from build123d import *

# Parameters (mm, degrees)
F1_DEPTH    = 55.5
F2_T        = 4
F2_T3_DEPTH = 63.5
F3_R        = 1.5
F3_R_2      = 5
F4_DEPTH    = 132
F6_START    = -4
F6_DEPTH    = 47.5


# Not quite as in the source:
# - a shell that OpenCascade refuses in one call is made with other operations: the cavity is built on its own and cut out


with BuildPart() as f1:
    # F0 (on Right) → F1 (new body)
    with BuildSketch(Plane.YZ):
        with BuildLine():
            Line((0, -55.0991142094), (0, 49.9008857906))
            Line((0, 49.9008857906), (-499, 49.9008857906))
            Line((-499, 49.9008857906), (-499, 20.9008857906))
            Line((-499, 20.9008857906), (-542, 20.9008857906))
            Line((-542, 20.9008857906), (-542, 49.9008857906))
            Line((-542, 49.9008857906), (-571, 49.9008857906))
            Line((-571, 49.9008857906), (-585.0227475166, 32.4236936867))
            ThreePointArc((-585.0227475166, 32.4236936867), (-589.1305886162, 10.6178817454), (-573.3100487518, -4.9409842581))
            Line((-573.3100487518, -4.9409842581), (0, -55.0991142094))
        make_face()
        with BuildLine():
            ThreePointArc((-267.5215016214, -12.4960653082), (-287.1014882349, 8.865775765), (-267.5215016214, 30.2276168381))
            ThreePointArc((-267.5215016214, 30.2276168381), (-265.5317159892, 30.3083194328), (-263.5430244658, 30.2040803041))
            Line((-263.5430244658, 30.2040803041), (-227.1501212267, 29.9887811395))
            ThreePointArc((-227.1501212267, 29.9887811395), (-226.7168570765, 29.9902909304), (-226.2836411156, 29.983655073))
            ThreePointArc((-226.2836411156, 29.983655073), (-210.3577454889, 23.0383320758), (-203.8081448594, 6.9456506758))
            ThreePointArc((-203.8081448594, 6.9456506758), (-210.3577454889, -9.1470307242), (-226.2836411156, -16.0923537213))
            ThreePointArc((-226.2836411156, -16.0923537213), (-228.8553111139, -16.012257226), (-231.40202441, -15.6459876318))
            Line((-231.40202441, -15.6459876318), (-267.5215016214, -12.4960653082))
        make_face(mode=Mode.SUBTRACT)
        with BuildLine():
            ThreePointArc((-112.6117591226, 30.1063306123), (-92.6236860119, 21.9492705288), (-84.3273722818, 2.0185938124))
            ThreePointArc((-84.3273722818, 2.0185938124), (-93.5072337014, -18.7521971721), (-115.0464908191, -25.9463626291))
            Line((-115.0464908191, -25.9463626291), (-137.5543760441, -23.8290179612))
            ThreePointArc((-137.5543760441, -23.8290179612), (-138.6707155639, -23.7473709318), (-139.7826970584, -23.6193970408))
            ThreePointArc((-139.7826970584, -23.6193970408), (-163.0572812206, 4.0202298169), (-137.871291965, 29.9300963926))
            ThreePointArc((-137.871291965, 29.9300963926), (-136.3367885283, 29.9845849808), (-134.8016741863, 29.9515129286))
            Line((-134.8016741863, 29.9515129286), (-112.6117591226, 30.1063306123))
        make_face(mode=Mode.SUBTRACT)
    extrude(amount=F1_DEPTH)

    # F2: shell of thickness 4, made by hand


with BuildPart() as f2_core1:
    # F2_t2: copy of F1
    add(f1.part)

    # the walls: a layer under each face that stays
    f2_faces = [f2_core1.faces().sort_by_distance(p)[0] for p in [
        (55.5, -295.1049872852, -2.5991142094),
        (27.75, -163.0392168361, 4.4361103036),
        (27.75, -126.3004334316, -24.8876902951),
        (27.75, -84.3538324473, 0.7996810334),
        (27.75, -123.7067166544, 30.0289217705),
        (27.75, -203.9075264936, 4.8077471556),
        (27.75, -245.3465728463, 30.0964307218),
        (27.75, -287.0090157551, 10.8550491528),
        (27.75, -249.4617630157, -14.07102647),
        (27.75, -589.1305886162, 10.6178817454),
        (27.75, -578.0113737583, 41.1622897387),
        (27.75, -556.5, 49.9008857906),
        (27.75, -520.5, 20.9008857906),
        (27.75, -499, 35.4008857906),
        (0, -295.1049872852, -2.5991142094),
        (27.75, -286.6550243759, -30.0200492338),
    ]]
    thicken(f2_faces, amount=-F2_T, mode=Mode.SUBTRACT)

    # F2_s4 → F2_t3 (cut)
    with BuildSketch(Plane.YZ.offset(-4)):
        Polygon((-499.04, 20.9408857906), (-499, 16.9008857906), (-495, 16.9008857906), (-495, 20.9008857906), align=None)
    extrude(amount=F2_T3_DEPTH, mode=Mode.SUBTRACT)


with BuildPart() as f1_1:
    add(f1.part)

    # what is left inside the walls is the cavity
    f2_cavity = [f2_core1.part.solids().sort_by_distance(p)[0] for p in [
        (51.46, -293.104987, -17.422261),
    ]]
    add(f2_cavity, mode=Mode.SUBTRACT)

    # F3 (on face) → F4 (cut)
    with BuildSketch(Plane.YZ.offset(55.5)):
        with Locations((-43.75, 33.9008857906)):
            Circle(F3_R)
        with Locations((-43.75, 22.9008857906)):
            Circle(F3_R)
        with Locations((-43.75, 11.9008857906)):
            Circle(F3_R)
        with Locations((-43.75, 0.9008857906)):
            Circle(F3_R)
        with Locations((-43.75, -10.0991142094)):
            Circle(F3_R)
        with Locations((-43.75, -21.0991142094)):
            Circle(F3_R)
        with Locations((-43.75, -43.2409264798)):
            Circle(F3_R)
        with Locations((-43.75, -32.0991142094)):
            Circle(F3_R)
        with Locations((-32, 0.9008857906)):
            Circle(F3_R)
        with Locations((-32, -10.0991142094)):
            Circle(F3_R)
        with Locations((-4.5, -43.2409264798)):
            Circle(F3_R)
        with Locations((-9, -43.2409264798)):
            Circle(F3_R)
        with Locations((-9, -32.0991142094)):
            Circle(F3_R)
        with Locations((-13.5, -32.0991142094)):
            Circle(F3_R)
        with Locations((-13.5, -43.2409264798)):
            Circle(F3_R)
        with Locations((-166.25, -21.1966199487)):
            Circle(F3_R)
        with Locations((-180.75, 22.9008857906)):
            Circle(F3_R)
        with Locations((-180.75, -21.2039937677)):
            Circle(F3_R)
        with Locations((-166.25, 22.9008857906)):
            Circle(F3_R)
        with Locations((-173.5, 33.9008857906)):
            Circle(F3_R)
        with Locations((-292.1831863405, 33.9008857906)):
            Circle(F3_R)
        with Locations((-292.1831863405, -18.4991142094)):
            Circle(F3_R)
        with Locations((-292.1831863405, 20.8008857906)):
            Circle(F3_R)
        with Locations((-292.1831863405, 7.7008857906)):
            Circle(F3_R)
        with Locations((-292.1831863405, -5.3991142094)):
            Circle(F3_R)
        with Locations((-576.1306285858, 17.892671749)):
            Circle(F3_R_2)
    extrude(amount=-F4_DEPTH, mode=Mode.SUBTRACT)

    # F5 (on face) → F6 (cut)
    with BuildSketch(Plane.YZ.offset(55.5).offset(F6_START)):
        Polygon((-77.8550534083, 42.2289334238), (-298.9033162594, 42.2289334238), (-298.9033162594, -20.6155626995), (-77.8550534083, -39.8928311294), align=None)
    extrude(amount=-F6_DEPTH, mode=Mode.SUBTRACT)


solid = f1_1.part
Read the model definition and answer for the solid it produces. Units are mm, in the model's axes. A direction names the side the tool comes from. Round coordinates to 2 decimals unless told otherwise and drop trailing zeros. Write each loop counter-clockwise with the first axis right and the second up, starting at its lowest first coordinate (ties: lowest second). Pieces come first, ordered by that corner, then holes.
Q1. Find section A-A on x = 31. Determine the outline of the cut face in (y, z).
Values:
outline: (-585.02, 32.42) arc R23.58 ccw to (-573.31, -4.94) - (0, -55.1) - (0, -51.08) - (-572.54, -0.99) arc R19.58 cw to (-581.9, 29.92) - (-569.08, 45.9) - (-542, 45.9) - (-542, 49.9) - (-571, 49.9) - close; (-542, 16.9) - (-495, 16.9) - (-495, 49.9) - (-499, 49.9) - (-499, 20.9) - (-542, 20.9) - close
Q2. Find section B-B on y = -147. Determine the outline of the cut face in (x, z).
Values:
outline: (0, -42.24) - (55.5, -42.24) - (55.5, -21.58) - (51.5, -21.58) - (51.5, -38.22) - (4, -38.22) - (4, -21.58) - (0, -21.58) - close; (0, 27.7) - (4, 27.7) - (4, 49.9) - (0, 49.9) - close; (51.5, 27.7) - (55.5, 27.7) - (55.5, 49.9) - (51.5, 49.9) - close
Q3. Find section C-C on y = -370.5. Determine the outline of the cut face in (x, z).
Values:
outline: (0, -22.68) - (55.5, -22.68) - (55.5, 49.9) - (51.5, 49.9) - (51.5, -18.67) - (4, -18.67) - (4, 49.9) - (0, 49.9) - close
Q4. Straight lines are drawn through the part: line 1 (X direction, y = -206, z = 31.5); line 2 (Z direction, x = 1.1, y = -13.5); line 3 (Z direction, x = 2.3, y = -166.25). For each, find the intervals that lie inside material, in ascending order.
Values:
line 1: x = 0 to 4, 51.5 to 55.5
line 2: z = -53.92 to -44.74, -41.74 to -33.6, -30.6 to 49.9
line 3: z = -40.55 to -22.7, -19.7 to 21.4, 24.4 to 49.9
Q5. A tool of negligible diameter and unlimited length cuts with its end or side. For faces 5 (the face through (27, -495, 33)), 6 (the face through (27, -518, 16.901)), 7 (the face through (27, -556, 49.901)), 8 (the face through (27, -520, 20.901)), from which of +Z, -Z, +X, -X, +Y, -Y can it reach the whole face along a straight path? Write none if from no direction.
Values:
face 5: +Z, +Y
face 6: +Y
face 7: +Z, +X, -X, +Y, -Y
face 8: +Z, +X, -X
Q6. The mould has two halves that part along Z. Classify faces 1 (the face through (27.418, -575.402, 38.023)), 2 (the face through (27.36, -290.67, -29.67)), 3 (the face through (1.972, -84.333, 1.437)), 4 (the face through (27.4, -577.9, 41.3)): released by +Z, released by -Z, zero draft, split by the parting line, or undercut.
Values:
face 1: undercut
face 2: released by -Z
face 3: undercut
face 4: released by +Z
Q7. Flat-ended cylindrical pins translate along their axes: P1, Ø3, axis at x = 19, y = -191, coming from the +Z side; P2, Ø2.5, axis at y = -173.5, z = 33.9, coming from the +X side; P3, Ø1, axis at x = 31.5, y = -431, coming from the -Z side; P4, Ø2, axis at x = 44.5, y = -289, coming from the -Z side. Find the tip coordinate at first contact, or state that the pin passes through.
Values:
P1: stops at z = -34.24
P2: passes through
P3: stops at z = -17.44
P4: stops at z = -29.9
